For this review, take the finished solid that the model builds, in its own axes (mm). Coordinates: 2 decimals unless noted, no trailing zeros. Order: outer loops, then holes, each group sorted by start corner. A loop starts at its lowest first (then second) coordinate and runs counter-clockwise, first axis right, second up. Notation, with made-up numbers: (52, 44.5) -> (65, 44.5) arc R22 cw to (65, 74.5) -> close; hole circle Ø9 at (23.5, 68.25). An arc over 180 degrees is marked (long way). Return JSON: item names as keys, results as strings. Group by question number.
Item 1: Take a section at B-B (z = 13.5). Count the separate pieces of the cut face and the enclosed holes in it, then the cut area to 3 significant figures.
Item 2: Take a section at D-D (x = 269.5). Write out the cut boundary in (y, z).
Item 3: Insertion check: pin 1 (2 mm diameter, centred on x = 237.5, y = 6, fed in from +Z); pin 2 (3 mm diameter, centred on x = 105.5, y = 6.5, fed in from +Z). Each pin has a flat end and moves straight along its axis. Give the tip position at first contact, or say it passes through.
Item 4: Take a section at A-A (y = 3.5). Write out the cut boundary in (x, z), then the cut area to 3 significant figures.
Item 5: Take a section at C-C (x = -199). Write out the cut boundary in (y, z).
Item 6: For line 1 along Z through (x, y) = (197, 8.5); line 2 along Z through (x, y) = (-550.5, 12), list the stretches that pass through material, from the lowest coordinate up.
```python
from build123d import *

# Parameters (mm, degrees)
F1_DEPTH = 19.05


with BuildPart() as f1:
    # F0 (on Front) → F1 (new body)
    with BuildSketch(Plane.XZ):
        with BuildLine():
            Line((-609.6, -44.45), (609.6, -44.45))
            Line((609.6, -44.45), (609.6, 44.45))
            Line((609.6, 44.45), (589.267039, 44.45))
            ThreePointArc((589.267039, 44.45), (527.05, -6.35), (464.832961, 44.45))
            Line((464.832961, 44.45), (438.681325, 44.45))
            ThreePointArc((438.681325, 44.45), (376.464286, -6.35), (314.247246, 44.45))
            Line((314.247246, 44.45), (288.095611, 44.45))
            ThreePointArc((288.095611, 44.45), (225.878571, -6.35), (163.661532, 44.45))
            Line((163.661532, 44.45), (137.509897, 44.45))
            ThreePointArc((137.509897, 44.45), (75.292857, -6.35), (13.075818, 44.45))
            Line((13.075818, 44.45), (-13.075818, 44.45))
            ThreePointArc((-13.075818, 44.45), (-75.292857, -6.35), (-137.509897, 44.45))
            Line((-137.509897, 44.45), (-163.661532, 44.45))
            ThreePointArc((-163.661532, 44.45), (-225.878571, -6.35), (-288.095611, 44.45))
            Line((-288.095611, 44.45), (-314.247246, 44.45))
            ThreePointArc((-314.247246, 44.45), (-376.464286, -6.35), (-438.681325, 44.45))
            Line((-438.681325, 44.45), (-464.832961, 44.45))
            ThreePointArc((-464.832961, 44.45), (-527.05, -6.35), (-589.267039, 44.45))
            Line((-589.267039, 44.45), (-609.6, 44.45))
            Line((-609.6, 44.45), (-609.6, -44.45))
        make_face()
    extrude(amount=-F1_DEPTH)


solid = f1.part
```
Findings below:
{
 "1": {"separate pieces": "9", "enclosed holes": "0", "area": "9,170 mm2"},
 "2": {"outline": "(0, -44.45) -> (19.05, -44.45) -> (19.05, 11) -> (0, 11) -> close"},
 "3": {"pin 1": "stops at z = -5.08", "pin 2": "stops at z = 2.13"},
 "4": {"outline": "(-609.6, -44.45) -> (609.6, -44.45) -> (609.6, 44.45) -> (589.27, 44.45) arc R63.5 cw to (464.83, 44.45) -> (438.68, 44.45) arc R63.5 cw to (314.25, 44.45) -> (288.1, 44.45) arc R63.5 cw to (163.66, 44.45) -> (137.51, 44.45) arc R63.5 cw to (13.08, 44.45) -> (-13.08, 44.45) arc R63.5 cw to (-137.51, 44.45) -> (-163.66, 44.45) arc R63.5 cw to (-288.1, 44.45) -> (-314.25, 44.45) arc R63.5 cw to (-438.68, 44.45) -> (-464.83, 44.45) arc R63.5 cw to (-589.27, 44.45) -> (-609.6, 44.45) -> close", "area": "70,500 mm2"},
 "5": {"outline": "(0, -44.45) -> (19.05, -44.45) -> (19.05, -0.38) -> (0, -0.38) -> close"},
 "6": {"line 1": "z = -44.45 to 0.6", "line 2": "z = -44.45 to -1.86"}
}
